Check sheet for the modelled part. Datum: model origin and axes. Units: mm. A direction names the side the tool comes from. Coordinates: 2 decimals unless noted, no trailing zeros. Order: outer loops, then holes, each group sorted by start corner. A loop starts at its lowest first (then second) coordinate and runs counter-clockwise, first axis right, second up.
1. Draft check along X on faces 1 (the flat face through (72, 77, -15)), 2 (the flat face through (78, 152.75, 15)), 3 (the flat face through (127.1, 20.6, 7.2)). Enter one of: released by +X, released by -X, zero draft, split by the parting line, or undercut.
2. Cross-section at B-B (y = 110.5). Enter the section's corners in (x, z), then the cut area to 4 significant figures.
3. Thickness scan on line 1 (Y direction, x = 19.5, z = 4); line 2 (X direction, y = 98.5, z = 2.5); line 3 (Z direction, x = 77.5, y = 84.5). Record the ranges inside material, lowest first.
4. Cross-section at C-C (x = 58.5). Enter the section's corners in (y, z).
5. Set-up check for faces 4 (the flat face through (-3.5, 73, 7)), 5 (the flat face through (3.4, 148.9, 14.8)): record each of +Z, -Z, +X, -X, +Y, -Y from which the full face is reachable in a straight line by a thin tool's end or side.
6. Cross-section at D-D (z = -6.5). Enter the section's corners in (x, y).
7. Gauge pin test, flat ends, axial feed: pin 1 Ø12 at (y, z) = (38.5, 11) entering from +X; pin 2 Ø1.5 at (x, y) = (71, 38.5) entering from +Z; pin 3 Ø10 at (y, z) = (29, -1) entering from +X. Record the tip position at first contact, or that the pin passes through.
8. Cross-section at A-A (z = 4). Enter the section's corners in (x, y), then the cut area to 3 significant figures.
Autodesk Fusion 360 part; units mm, degrees
sketch "BoardOutline" plane through (0, 0, 0) normal (0, 0, 1) x (1, 0, 0)
  line L0 (0, 0) -> (101.5, 0)
  line L1 (147, 45.5) -> (147, 152.5)
  line L2 (147, 152.5) -> (7.5, 152.5)
  line L3 (0, 145) -> (0, 0)
  line L4 (7.5, 152.5) -> (0, 145)
  line L5 (147, 45.5) -> (101.5, 0)
  line L6 (7.5, 152.5) -> (7.5, 0) construction
  line L7 (147, 45.5) -> (0, 45.5) construction
  line L8 (101.5, 0) -> (101.5, 152.5) construction
  circle A0 centre (101.5, 45.5) radius 2
  line L9 (0, 145) -> (147, 145) construction
  circle A1 centre (7.5, 145) radius 2
  circle A2 centre (41.5, 145) radius 2
  circle A3 centre (134.5, 145) radius 2
  line L10 (134.5, 152.5) -> (134.5, 33) construction
  circle A4 centre (134.5, 90) radius 2
  circle A5 centre (134.5, 90) radius 2
  circle A6 centre (134.5, 90) radius 2
  circle A7 centre (41.5, 90) radius 2
  circle A8 centre (7.5, 133.5) radius 1.5
  circle A9 centre (7.5, 124.5) radius 1
  circle A10 centre (7.5, 87.5) radius 1
  circle A11 centre (26.5, 124.5) radius 1
  circle A12 centre (26.5, 87.5) radius 1
  circle A13 centre (7.5, 73.5) radius 2
  circle A14 centre (7.5, 7.5) radius 2
  circle A15 centre (131.0677, 63.4488) radius 6 construction
  line L11 (16.5, 0) -> (23.5, 0) construction
  line L12 (23.5, 0) -> (23.5, 13.6837) construction
  line L13 (23.5, 13.6837) -> (16.5, 13.6837) construction
  line L14 (16.5, 13.6837) -> (16.5, 0) construction
  line L15 (96, 0) -> (26, 0) construction
  line L16 (26, 0) -> (26, 82.5) construction
  line L17 (26, 82.5) -> (96, 82.5) construction
  line L18 (96, 82.5) -> (96, 0) construction
  line L19 (55.5, 0) -> (55.5, 10) construction
  line L20 (55.5, 10) -> (45.5, 10) construction
  line L21 (45.5, 10) -> (45.5, 0) construction
  line L22 (45.5, 0) -> (55.5, 0) construction
  line L23 (101.5, 45.5) -> (96, 45.5) construction
  line L24 (55.5, 0) -> (96, 0) construction
  line L25 (51, 130) -> (125, 130) construction
  line L26 (125, 130) -> (125, 105) construction
  line L27 (125, 105) -> (51, 105) construction
  line L28 (51, 105) -> (51, 130) construction
  point P0 (147, 0)
  point P1 (0, 152.5)
  point P2 (7.5, 145)
  point P3 (7.5, 73.5)
  dimension "d1" = 147
  dimension "d2" = 152.5
  dimension "d3" = 7.5
  dimension "d4" = 7.5
  dimension "d5" = 45.5
  dimension "d6" = 45.5
  dimension "d8" = 4
  dimension "d12" = 4
  dimension "d13" = 4
  dimension "d14" = 4
  dimension "d15" = 4
  dimension "d16" = 4
  dimension "d17" = 4
  dimension "d18" = 4
  dimension "d20" = 3
  dimension "d23" = 2
  dimension "d24" = 2
  dimension "d25" = 2
  dimension "d26" = 2
  dimension "d27" = 4
  dimension "d28" = 4
  dimension "d31" = 12
  dimension "d34" = 7
  dimension "d35" = 70
  dimension "d36" = 82.5
  dimension "d39" = 10
  dimension "d40" = 5.5
  dimension "d41" = 93
  dimension "d43" = 55
  dimension "d46" = 34
sketch "CasingOutline" plane through (0, 0, 0) normal (0, 0, 1) x (1, 0, 0)
  line L0 (-0.25, -0.25) -> (101.75, -0.25)
  line L1 (147.25, 45.25) -> (147.25, 152.75)
  line L2 (147.25, 152.75) -> (7.25, 152.75)
  line L3 (-0.25, 145.25) -> (-0.25, -0.25)
  line L4 (-3.5, -3.5) -> (103, -3.5)
  line L5 (150.5, 44) -> (150.5, 156)
  line L6 (150.5, 156) -> (5.5, 156)
  line L7 (-3.5, 147) -> (-3.5, -3.5)
  line L8 (147, 152.5) -> (7.5, 152.5)
  line L9 (147.25, 45.25) -> (101.75, -0.25)
  line L10 (-0.25, 145.25) -> (7.25, 152.75)
  line L11 (5.5, 156) -> (-3.5, 147)
  line L12 (150.5, 44) -> (103, -3.5)
  point P0 (147.25, -0.25)
  point P1 (-0.25, 152.75)
  point P2 (150.5, -3.5)
  point P3 (-3.5, 156)
  dimension "d50" = 147.5
  dimension "d51" = 153
  dimension "d52" = 3.25
  dimension "d53" = 3.25
  dimension "d55" = 3.25
  dimension "d56" = 3.25
  dimension "d57" = 45.5
  dimension "d58" = 45.5
  dimension "d59" = 7.5
  dimension "d60" = 7.5
  dimension "d61" = 9
  dimension "d62" = 9
  dimension "d63" = 47.5
  dimension "d64" = 47.5
extrude "Extrude1" add sketch "CasingOutline" against normal blind 15 contours L0 L1 L2 L3 L9 L10 | L4 L5 L6 L7 L11 L12
extrude "Extrude2" add sketch "CasingOutline" along normal blind 30
equation "d4 = d3"
equation "d6 = d5"
equation "d58 = d57"
equation "d60 = d59"
equation "d62 = d61"
equation "d64 = d63"
Data:
1. face 1: zero draft
1. face 2: undercut
1. face 3: released by +X
2. outline: (-3.5, -15) - (150.5, -15) - (150.5, 30) - (147.25, 30) - (147.25, 0) - (-0.25, 0) - (-0.25, 30) - (-3.5, 30) - close
2. area: 2,505 mm2
3. line 1: y = -3.5 to -0.25, 152.75 to 156
3. line 2: x = -3.5 to -0.25, 147.25 to 150.5
3. line 3: z = -15 to 0
4. outline: (-3.5, -15) - (156, -15) - (156, 30) - (152.75, 30) - (152.75, 0) - (-0.25, 0) - (-0.25, 30) - (-3.5, 30) - close
5. face 4: +Z, -Z, -X, +Y, -Y
5. face 5: +Z
6. outline: (-3.5, -3.5) - (103, -3.5) - (150.5, 44) - (150.5, 156) - (5.5, 156) - (-3.5, 147) - close
7. pin 1: stops at x = 150.5
7. pin 2: stops at z = 0
7. pin 3: stops at x = 140.5
8. outline: (-3.5, -3.5) - (103, -3.5) - (150.5, 44) - (150.5, 156) - (5.5, 156) - (-3.5, 147) - close; hole (-0.25, -0.25) - (101.75, -0.25) - (147.25, 45.25) - (147.25, 152.75) - (7.25, 152.75) - (-0.25, 145.25) - close
8. area: 1,890 mm2
